Print and shaded views of the part. All mm, measured from the part's lowest x, y and z. Give positions to 0.01 mm unless a question says otherwise; leave off trailing zeros. Write each loop counter-clockwise with the first axis right and the second up, starting at its lowest first coordinate (ties: lowest second). Pieces come first, ordered by that corner, then holes. Notation, with made-up numbers: (76, -26) - (115, -26) arc R28 ccw to (115, -1) - close; hole circle Ø10 at (16.5, 26.5). An arc over 180 degrees is marked (long way). Use one line per item in the form item = value. Start each with the question number.
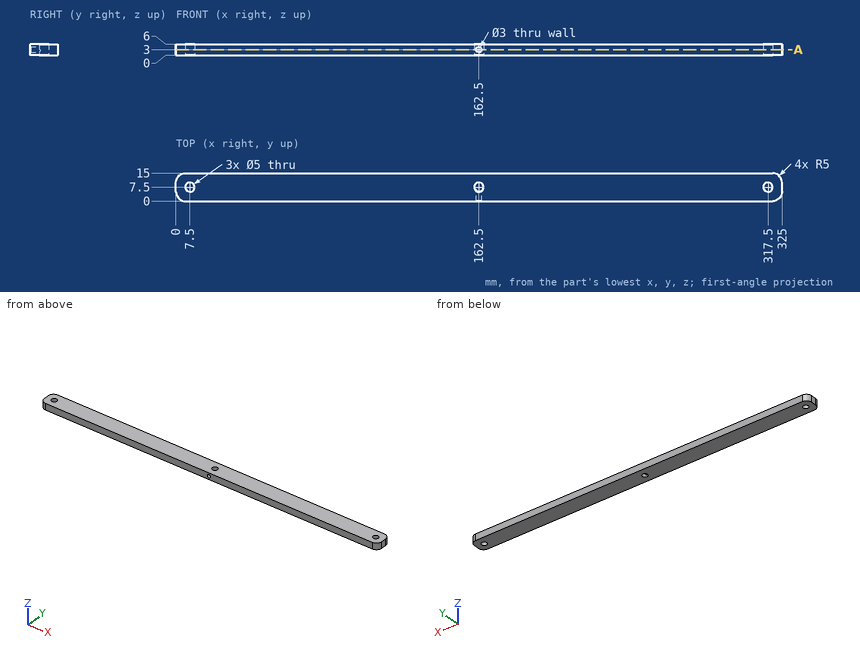
(1) Pin check, flat tip, straight feed: pin 1 Ø2 at (y, z) = (2, 3.5) entering from +X. Stop position of the tip, or through.
(2) Cut at A-A, the plane z = 3. Give the cut face in (x, y), then the cut area to 3 significant figures.
(3) Wall check: line 1 (Z direction, x = 162.5, y = 1.4); line 2 (X direction, y = 9.25, z = 5); line 3 (Y direction, x = 317.5, z = 2.6). Give the ranges that are in metal, low to high. Write a range as from..to.
Solution:
q1.pin_1 = 324.58
q2.outline = (0, 5) arc R5 ccw to (5, 0) - (161, 0) - (161, 5.5) arc R2.5 cw (long way) to (164, 5.5) - (164, 0) - (320, 0) arc R5 ccw to (325, 5) - (325, 10) arc R5 ccw to (320, 15) - (5, 15) arc R5 ccw to (0, 10) - close; hole circle Ø5 at (7.5, 7.5); hole circle Ø5 at (317.5, 7.5)
q2.area = 4,780 mm2
q3.line_1 = 0..1.5, 4.5..6
q3.line_2 = 0..5.71, 9.29..160.71, 164.29..315.71, 319.29..325
q3.line_3 = 0..5, 10..15
